Check sheet for the modelled part. Datum: model origin and axes. Units: mm. Give positions to 0.01 mm unless a question says otherwise; leave off trailing zeros. Write each loop counter-clockwise with the first axis right and the second up, starting at its lowest first coordinate (ties: lowest second). Pieces come first, ordered by that corner, then holes. Notation, with made-up numbers: M 72,53 L 96,53 A17 cw 96,66 Z; hole C 38.5,2.25 d9. An arc over 180 degrees is marked long. One line per item, written item: value. Start each with the question number.
from build123d import *

# Parameters (mm, degrees)
SKETCH1_W           = 170
SKETCH1_H           = 106
BOSS_EXTRUDE1_DEPTH = 5
CUT_EXTRUDE2_REACH  = 202.402


with BuildPart() as part:
    # Sketch1 → Boss-Extrude1 (new body)
    with BuildSketch(Plane(origin=(0, 0, 0), x_dir=(1, 0, 0), z_dir=(0, 1, 0))):
        with Locations((85, 53)):
            Rectangle(SKETCH1_W, SKETCH1_H)
    extrude(amount=BOSS_EXTRUDE1_DEPTH)

    # Sketch2 → Cut-Extrude2 (cut, up to next)
    with BuildSketch(Plane(origin=(0, 5, 0), x_dir=(1, 0, 0), z_dir=(0, 1, 0)), mode=Mode.PRIVATE) as cut_extrude2_sk1:
        with BuildLine():
            Line((10, 98.605263158), (160, 98.605263158))
            ThreePointArc((160, 98.605263158), (162.605263158, 96), (160, 93.394736842))
            Line((160, 93.394736842), (10, 93.394736842))
            ThreePointArc((10, 93.394736842), (7.394736842, 96), (10, 98.605263158))
        make_face()
    cut_extrude2_tool1 = extrude(cut_extrude2_sk1.sketch, amount=-CUT_EXTRUDE2_REACH, mode=Mode.PRIVATE) & part.part
    # Sketch2 → Cut-Extrude2 (cut, up to next)
    with BuildSketch(Plane(origin=(0, 5, 0), x_dir=(1, 0, 0), z_dir=(0, 1, 0)), mode=Mode.PRIVATE) as cut_extrude2_sk2:
        with BuildLine():
            Line((10, 89.105263158), (160, 89.105263158))
            ThreePointArc((160, 89.105263158), (162.605263158, 86.5), (160, 83.894736842))
            Line((160, 83.894736842), (10, 83.894736842))
            ThreePointArc((10, 83.894736842), (7.394736842, 86.5), (10, 89.105263158))
        make_face()
    cut_extrude2_tool2 = extrude(cut_extrude2_sk2.sketch, amount=-CUT_EXTRUDE2_REACH, mode=Mode.PRIVATE) & part.part
    # Sketch2 → Cut-Extrude2 (cut, up to next)
    with BuildSketch(Plane(origin=(0, 5, 0), x_dir=(1, 0, 0), z_dir=(0, 1, 0)), mode=Mode.PRIVATE) as cut_extrude2_sk3:
        with BuildLine():
            Line((10, 79.605263158), (160, 79.605263158))
            ThreePointArc((160, 79.605263158), (162.605263158, 77), (160, 74.394736842))
            Line((160, 74.394736842), (10, 74.394736842))
            ThreePointArc((10, 74.394736842), (7.394736842, 77), (10, 79.605263158))
        make_face()
    cut_extrude2_tool3 = extrude(cut_extrude2_sk3.sketch, amount=-CUT_EXTRUDE2_REACH, mode=Mode.PRIVATE) & part.part
    # Sketch2 → Cut-Extrude2 (cut, up to next)
    with BuildSketch(Plane(origin=(0, 5, 0), x_dir=(1, 0, 0), z_dir=(0, 1, 0)), mode=Mode.PRIVATE) as cut_extrude2_sk4:
        with BuildLine():
            Line((10, 70.105263158), (160, 70.105263158))
            ThreePointArc((160, 70.105263158), (162.605263158, 67.5), (160, 64.894736842))
            Line((160, 64.894736842), (10, 64.894736842))
            ThreePointArc((10, 64.894736842), (7.394736842, 67.5), (10, 70.105263158))
        make_face()
    cut_extrude2_tool4 = extrude(cut_extrude2_sk4.sketch, amount=-CUT_EXTRUDE2_REACH, mode=Mode.PRIVATE) & part.part
    # Sketch2 → Cut-Extrude2 (cut, up to next)
    with BuildSketch(Plane(origin=(0, 5, 0), x_dir=(1, 0, 0), z_dir=(0, 1, 0)), mode=Mode.PRIVATE) as cut_extrude2_sk5:
        with BuildLine():
            Line((10, 60.605263158), (160, 60.605263158))
            ThreePointArc((160, 60.605263158), (162.605263158, 58), (160, 55.394736842))
            Line((160, 55.394736842), (10, 55.394736842))
            ThreePointArc((10, 55.394736842), (7.394736842, 58), (10, 60.605263158))
        make_face()
    cut_extrude2_tool5 = extrude(cut_extrude2_sk5.sketch, amount=-CUT_EXTRUDE2_REACH, mode=Mode.PRIVATE) & part.part
    # Sketch2 → Cut-Extrude2 (cut, up to next)
    with BuildSketch(Plane(origin=(0, 5, 0), x_dir=(1, 0, 0), z_dir=(0, 1, 0)), mode=Mode.PRIVATE) as cut_extrude2_sk6:
        with BuildLine():
            Line((10, 51.105263158), (160, 51.105263158))
            ThreePointArc((160, 51.105263158), (162.605263158, 48.5), (160, 45.894736842))
            Line((160, 45.894736842), (10, 45.894736842))
            ThreePointArc((10, 45.894736842), (7.394736842, 48.5), (10, 51.105263158))
        make_face()
    cut_extrude2_tool6 = extrude(cut_extrude2_sk6.sketch, amount=-CUT_EXTRUDE2_REACH, mode=Mode.PRIVATE) & part.part
    # Sketch2 → Cut-Extrude2 (cut, up to next)
    with BuildSketch(Plane(origin=(0, 5, 0), x_dir=(1, 0, 0), z_dir=(0, 1, 0)), mode=Mode.PRIVATE) as cut_extrude2_sk7:
        with BuildLine():
            Line((10, 41.605263158), (160, 41.605263158))
            ThreePointArc((160, 41.605263158), (162.605263158, 39), (160, 36.394736842))
            Line((160, 36.394736842), (10, 36.394736842))
            ThreePointArc((10, 36.394736842), (7.394736842, 39), (10, 41.605263158))
        make_face()
    cut_extrude2_tool7 = extrude(cut_extrude2_sk7.sketch, amount=-CUT_EXTRUDE2_REACH, mode=Mode.PRIVATE) & part.part
    # Sketch2 → Cut-Extrude2 (cut, up to next)
    with BuildSketch(Plane(origin=(0, 5, 0), x_dir=(1, 0, 0), z_dir=(0, 1, 0)), mode=Mode.PRIVATE) as cut_extrude2_sk8:
        with BuildLine():
            Line((10, 32.105263158), (160, 32.105263158))
            ThreePointArc((160, 32.105263158), (162.605263158, 29.5), (160, 26.894736842))
            Line((160, 26.894736842), (10, 26.894736842))
            ThreePointArc((10, 26.894736842), (7.394736842, 29.5), (10, 32.105263158))
        make_face()
    cut_extrude2_tool8 = extrude(cut_extrude2_sk8.sketch, amount=-CUT_EXTRUDE2_REACH, mode=Mode.PRIVATE) & part.part
    # Sketch2 → Cut-Extrude2 (cut, up to next)
    with BuildSketch(Plane(origin=(0, 5, 0), x_dir=(1, 0, 0), z_dir=(0, 1, 0)), mode=Mode.PRIVATE) as cut_extrude2_sk9:
        with BuildLine():
            Line((10, 22.605263158), (160, 22.605263158))
            ThreePointArc((160, 22.605263158), (162.605263158, 20), (160, 17.394736842))
            Line((160, 17.394736842), (10, 17.394736842))
            ThreePointArc((10, 17.394736842), (7.394736842, 20), (10, 22.605263158))
        make_face()
    cut_extrude2_tool9 = extrude(cut_extrude2_sk9.sketch, amount=-CUT_EXTRUDE2_REACH, mode=Mode.PRIVATE) & part.part
    # Sketch2 → Cut-Extrude2 (cut, up to next)
    with BuildSketch(Plane(origin=(0, 5, 0), x_dir=(1, 0, 0), z_dir=(0, 1, 0)), mode=Mode.PRIVATE) as cut_extrude2_sk10:
        with BuildLine():
            Line((10, 13.105263158), (160, 13.105263158))
            ThreePointArc((160, 13.105263158), (162.605263158, 10.5), (160, 7.894736842))
            Line((160, 7.894736842), (10, 7.894736842))
            ThreePointArc((10, 7.894736842), (7.394736842, 10.5), (10, 13.105263158))
        make_face()
    cut_extrude2_tool10 = extrude(cut_extrude2_sk10.sketch, amount=-CUT_EXTRUDE2_REACH, mode=Mode.PRIVATE) & part.part
    add(cut_extrude2_tool1.solids().sort_by_distance((85, 5, -96))[0], mode=Mode.SUBTRACT)
    add(cut_extrude2_tool2.solids().sort_by_distance((85, 5, -86.5))[0], mode=Mode.SUBTRACT)
    add(cut_extrude2_tool3.solids().sort_by_distance((85, 5, -77))[0], mode=Mode.SUBTRACT)
    add(cut_extrude2_tool4.solids().sort_by_distance((85, 5, -67.5))[0], mode=Mode.SUBTRACT)
    add(cut_extrude2_tool5.solids().sort_by_distance((85, 5, -58))[0], mode=Mode.SUBTRACT)
    add(cut_extrude2_tool6.solids().sort_by_distance((85, 5, -48.5))[0], mode=Mode.SUBTRACT)
    add(cut_extrude2_tool7.solids().sort_by_distance((85, 5, -39))[0], mode=Mode.SUBTRACT)
    add(cut_extrude2_tool8.solids().sort_by_distance((85, 5, -29.5))[0], mode=Mode.SUBTRACT)
    add(cut_extrude2_tool9.solids().sort_by_distance((85, 5, -20))[0], mode=Mode.SUBTRACT)
    add(cut_extrude2_tool10.solids().sort_by_distance((85, 5, -10.5))[0], mode=Mode.SUBTRACT)


solid = part.part
1) Draft check along Z on faces 1 (the cylindrical face through (162.605, 2.535, -10.557)), 2 (the flat face through (0, 2, -52)), 3 (the cylindrical face through (7.395, 2.535, -48.443)), 4 (the flat face through (84, 2, 0)). Enter one of: released by +Z, released by -Z, zero draft, split by the parting line, or undercut.
2) Cross-section at B-B (x = 97.5). State how many separate pieces and enclosed holes the cut face has, plus the area to 3 significant figures.
3) Cross-section at A-A (z = -86.5). Record the boundary of the cut face in (x, y).
4) Material ranges on L1, parallel to X at y = 1.7, z = -10.5; L2, parallel to X at y = 3.8, z = -28, recorded low to high. Write a range as from..to.
Data:
1. face 1: undercut
1. face 2: zero draft
1. face 3: undercut
1. face 4: released by +Z
2. separate pieces: 11
2. enclosed holes: 0
2. area: 269 mm2
3. outline: M 0,0 L 7.39,0 L 7.39,5 L 0,5 Z; M 162.61,0 L 170,0 L 170,5 L 162.61,5 Z
4. L1: x = 0..7.39, 162.61..170
4. L2: x = 0..7.87, 162.13..170
